Geometry check sheet. Reference: drawing and pictorial views, mm from the part's lowest x, y, z. A direction names the side the tool comes from. Give positions to 0.01 mm unless a question says otherwise; leave off trailing zeros. Order: outer loops, then holes, each group sorted by start corner. A loop starts at its lowest first (then second) coordinate and runs counter-clockwise, first axis right, second up.
Item 1: Sectioned sample at D-D on y = 7.5. Record the boundary of the cut face in (x, z).
Item 2: Sectioned sample at B-B on z = 9.5. Record the boundary of the cut face in (x, y), and give its area (3 significant figures).
Item 3: Sectioned sample at A-A on x = 12. Record the boundary of the cut face in (y, z).
Item 4: Sectioned sample at C-C on z = 14.25. Record the boundary of the cut face in (x, y), and give its area (3 significant figures).
Item 5: Access from +Z, -Z, +X, -X, +Y, -Y to the whole of each face (thin tool, end or side, straight path). Record for the marked faces 1, 2 and 3.
Item 6: Release check for a two-part mould opening along Z. For the marked faces 4, 5, 6 and 7 record: released by +Z, released by -Z, zero draft, split by the parting line, or undercut.
Item 7: Material ranges on line 1 along X through (y, z) = (11.75, 14); line 2 along Z through (x, y) = (25, 6.25); line 3 along X through (y, z) = (12.5, 9), recorded low to high.
Item 8: Gauge pin test, flat ends, axial feed: P1, Ø5, axis at x = 27, y = 3, coming from the -Z side; P2, Ø1.4, axis at x = 16, z = 2.5, coming from the -Y side. Record the tip position at first contact, or that the pin passes through.
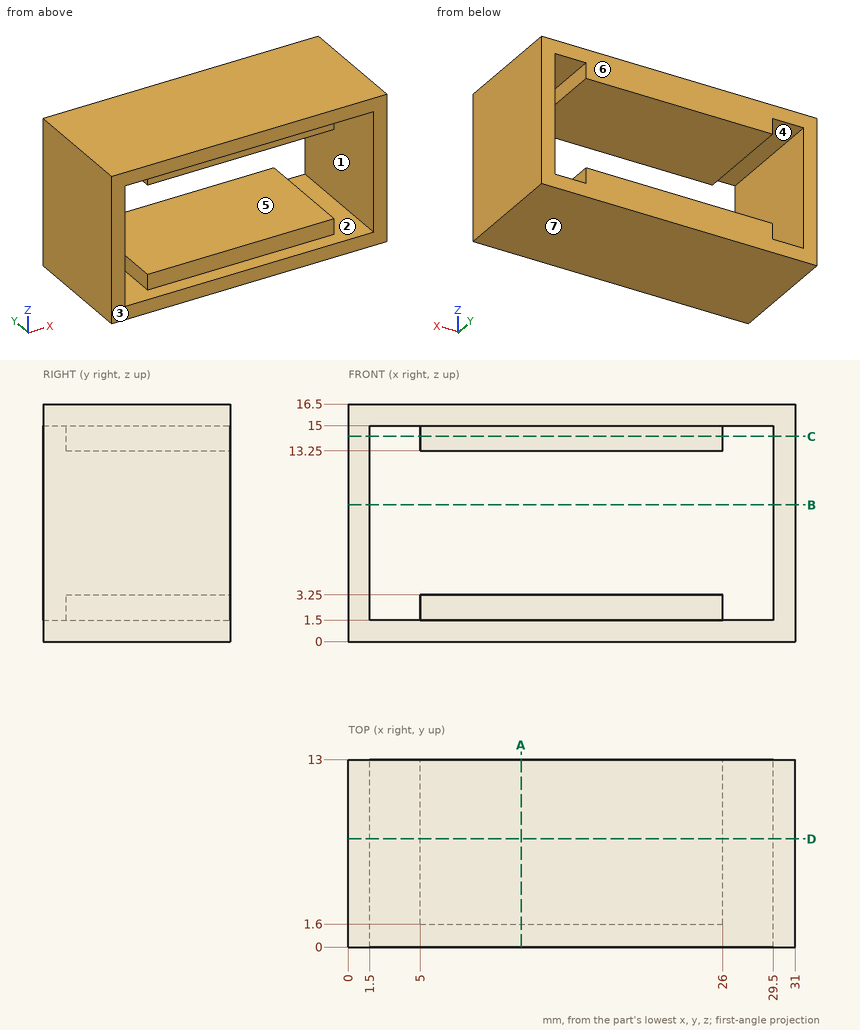
Report:
1. outline: (0, 0) - (31, 0) - (31, 16.5) - (0, 16.5) - close; hole (1.5, 1.5) - (5, 1.5) - (5, 3.25) - (26, 3.25) - (26, 1.5) - (29.5, 1.5) - (29.5, 15) - (26, 15) - (26, 13.25) - (5, 13.25) - (5, 15) - (1.5, 15) - close
2. outline: (0, 0) - (1.5, 0) - (1.5, 13) - (0, 13) - close; (29.5, 0) - (31, 0) - (31, 13) - (29.5, 13) - close
2. area: 39.0 mm2
3. outline: (0, 0) - (13, 0) - (13, 3.25) - (1.6, 3.25) - (1.6, 1.5) - (0, 1.5) - close; (0, 15) - (1.6, 15) - (1.6, 13.25) - (13, 13.25) - (13, 16.5) - (0, 16.5) - close
4. outline: (0, 0) - (1.5, 0) - (1.5, 13) - (0, 13) - close; (5, 1.6) - (26, 1.6) - (26, 13) - (5, 13) - close; (29.5, 0) - (31, 0) - (31, 13) - (29.5, 13) - close
4. area: 278 mm2
5. face 1: +Y, -Y
5. face 2: -Y
5. face 3: +Z, -Z, +X, -X, -Y
6. face 4: undercut
6. face 5: undercut
6. face 6: zero draft
6. face 7: released by -Z
7. line 1: x = 0 to 1.5, 5 to 26, 29.5 to 31
7. line 2: z = 0 to 3.25, 13.25 to 16.5
7. line 3: x = 0 to 1.5, 29.5 to 31
8. P1: stops at z = 0
8. P2: stops at y = 1.6
